Part model, mm, in its own coordinate system. Face numbers are marked on the shaded views. A direction names the side the tool comes from. Give positions to 0.01 mm unless a question says otherwise; leave off trailing zeros. Write each loop counter-clockwise with the first axis right and the second up, starting at its lowest first coordinate (ties: lowest second). Pieces come first, ordered by that corner, then holes. Notation, with made-up numbers: M 48,82 L 59,82 A19 ccw 59,91 Z; hole C 6,-40 d10. An arc over 180 degrees is marked long. Use a Markdown table: item, result.
```python
from build123d import *

# Parameters (mm, degrees)
SKETCH_2_R      = 2.5
EXTRUDE_1_DEPTH = 2
SKETCH_3_R      = 2.5
EXTRUDE_2_DEPTH = 2
FILLET_1_R      = 2


with BuildPart() as part:
    # 草图2 → 凸台-拉伸1 (new body)
    with BuildSketch(Plane(origin=(0, 0, 0), x_dir=(1, 0, 0), z_dir=(0, 1, 0))):
        with BuildLine():
            Line((0, 0), (16, 0))
            Line((16, 0), (16, 12))
            ThreePointArc((16, 12), (8, 20), (0, 12))
            Line((0, 12), (0, 0))
        make_face()
        with Locations(Location((8, 12, 0), (0, 0, 270))):
            Circle(SKETCH_2_R, mode=Mode.SUBTRACT)
    extrude(amount=EXTRUDE_1_DEPTH)

    # 草图3 → 凸台-拉伸2 (add)
    with BuildSketch(Plane.XY):
        with BuildLine():
            Line((0, 0), (16, 0))
            Line((16, 0), (16, 12))
            ThreePointArc((16, 12), (8, 20), (0, 12))
            Line((0, 12), (0, 0))
        make_face()
        with Locations((8, 12)):
            Circle(SKETCH_3_R, mode=Mode.SUBTRACT)
    extrude(amount=-EXTRUDE_2_DEPTH)

    # 圆角1
    fillet_1_edges = [part.edges().sort_by_distance(p)[0] for p in [
        (8, 2, -2),
        (8, 0, 0),
    ]]
    fillet(fillet_1_edges, radius=FILLET_1_R)


solid = part.part
```
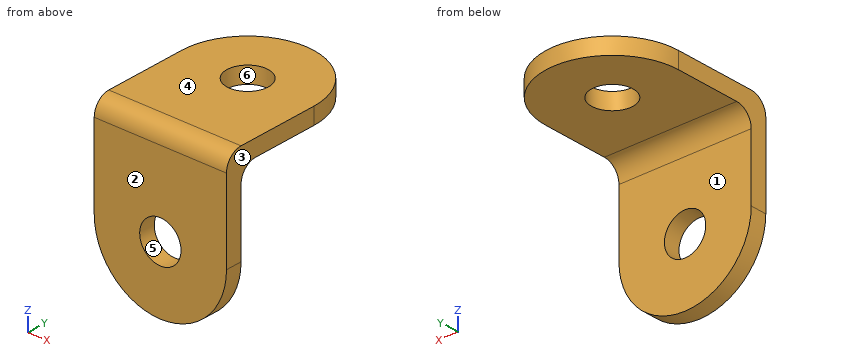
1. Two-plate mould, pull along X, no slides. Class the marked faces 3, 4, 5 and 6: released by +X, released by -X, zero draft, split by the parting line, or undercut.
Findings below:
| item | result |
|---|---|
| face 3 | released by +X |
| face 4 | zero draft |
| face 5 | undercut |
| face 6 | undercut |
2. Drop a flat-ended pin along its axis: P1, Ø1, axis at x = 12.5, y = 15.5, coming from the -Z side. Give the stop position or say it passes through.
Findings below:
| item | result |
|---|---|
| P1 | z = -2 |
3. Cut at A-A, the plane x = 8. Give the cut face in (y, z).
Findings below:
| item | result |
|---|---|
| outline | M 0,-20 L 2,-20 L 2,-14.5 L 0,-14.5 Z; M 0,-9.5 L 2,-9.5 L 2,-4 A2 cw 4,-2 L 9.5,-2 L 9.5,0 L 2,0 A2 ccw 0,-2 Z; M 14.5,-2 L 20,-2 L 20,0 L 14.5,0 Z |
4. Drill centre lines: L1, parallel to X at y = 1, z = -12; L2, parallel to Z at x = 7.25, y = 15.75; L3, parallel to Y at x = 12.5, z = -15.25. Where is each one in solid material? Low to high.
Findings below:
| item | result |
|---|---|
| L1 | 0 to 5.5, 10.5 to 16 |
| L2 | -2 to 0 |
| L3 | 0 to 2 |
5. Cut at B-B, the plane z = -11.5. Give the cut face in (x, y).
Findings below:
| item | result |
|---|---|
| outline | M 0,0 L 5.55,0 L 5.55,2 L 0,2 Z; M 10.45,0 L 16,0 L 16,2 L 10.45,2 Z |
6. Cut at C-C, the plane y = 13.25. Give the cut face in (x, z), then the cut area to 3 significant figures.
Findings below:
| item | result |
|---|---|
| outline | M 0.1,-2 L 5.83,-2 L 5.83,0 L 0.1,0 Z; M 10.17,-2 L 15.9,-2 L 15.9,0 L 10.17,0 Z |
| area | 22.9 mm2 |
7. Tool access for the marked faces 1 and 2: list every direction of +Z, -Z, +X, -X, +Y, -Y with a clear straight run to the whole face (end or side of a thin tool).
Findings below:
| item | result |
|---|---|
| face 1 | -Z, +X, -X, +Y |
| face 2 | +Z, -Z, +X, -X, -Y |
8. Cut at D-D, the plane x = 12. Give the cut face in (y, z).
Findings below:
| item | result |
|---|---|
| outline | M 0,-18.93 L 2,-18.93 L 2,-4 A2 cw 4,-2 L 18.93,-2 L 18.93,0 L 2,0 A2 ccw 0,-2 Z |
